```python
from build123d import *

# Parameters (mm, degrees)
F0_W     = 63.5
F0_H     = 19.05
F1_DEPTH = 558.8
F2_SIZE  = 3.175
F3_W     = 12.7
F3_H     = 6.35
F4_DEPTH = 558.801


with BuildPart() as f1:
    # F0 (on Top) → F1 (new body)
    with BuildSketch(Plane.XY):
        with Locations((31.75, 9.525)):
            Rectangle(F0_W, F0_H)
    extrude(amount=F1_DEPTH)

    # F2
    f2_edges = [f1.edges().sort_by_distance(p)[0] for p in [
        (0, 19.05, 279.4),
        (63.5, 19.05, 279.4),
        (31.75, 19.05, 0),
        (31.75, 19.05, 558.8),
    ]]
    chamfer(f2_edges, length=F2_SIZE)

    # F3 (on face) → F4 (cut, through all)
    with BuildSketch(Plane(origin=(0, 0, 0), x_dir=(1, 0, 0), z_dir=(0, 0, -1))):
        with Locations((57.15, -7.9375)):
            Rectangle(F3_W, F3_H)
    extrude(amount=-F4_DEPTH, mode=Mode.SUBTRACT)


solid = f1.part
```
The model under review builds one solid part; all positions refer to its coordinate system, in mm. Round coordinates to 2 decimals unless told otherwise and drop trailing zeros. Write each loop counter-clockwise with the first axis right and the second up, starting at its lowest first coordinate (ties: lowest second). Pieces come first, ordered by that corner, then holes. Notation, with made-up numbers: M 23.5,33 L 82.5,33 A11 cw 82.5,46 Z; hole C -25,38.5 d1. An arc over 180 degrees is marked long. Use CSV: the item, a comma, the result in double quotes. Start each with the question number.
(1) We need section B-B, the plane y = 8.25. State the section outline as (x, z) points, then the cut area to 3 significant figures.
(2) For line 1 along Y through (x, z) = (56, 432); line 2 along X through (y, z) = (6.75, 266.5); line 3 along Y through (x, z) = (61, 33) (1 decimal), list the stretches that pass through material, from the lowest coordinate up.
(3) The part is to be moulded in two halves that separate along Y. For faces 1 (the face through (31, 8, 0)), 2 (the face through (57, 4.762, 275)), 3 (the face through (57, 11.112, 275)), 4 (the face through (31, 0, 275)), say which applies: +Y half, -Y half, draft (parallel to the pull), parting line (faces both ways), or undercut.
Findings:
1,outline,"M 0,0 L 50.8,0 L 50.8,558.8 L 0,558.8 Z"
1,area,"28,400 mm^2"
2,line 1,"0 to 4.76, 11.11 to 19.05"
2,line 2,"0 to 50.8"
2,line 3,"0 to 4.8, 11.1 to 18.4"
3,face 1,"draft"
3,face 2,"undercut"
3,face 3,"undercut"
3,face 4,"-Y half"
